The model under review builds one solid part; all positions refer to its coordinate system, in mm. Face numbers are marked on the shaded views. Coordinates: 2 decimals unless noted, no trailing zeros. Order: outer loops, then holes, each group sorted by start corner. A loop starts at its lowest first (then second) coordinate and runs counter-clockwise, first axis right, second up. Notation, with made-up numbers: (61.5, -17.5) -> (66.5, -17.5) arc R5 ccw to (66.5, -10.5) -> close; hole circle Ø9 at (-29.75, 88.5). An arc over 180 degrees is marked (long way). Put each result on its own line as item: value.
Autodesk Inventor part; units mm, degrees
ref_plane "YZ Plane" through (0, 0, 0) normal (1, 0, 0) x (0, 1, 0)
ref_plane "XZ Plane" through (0, 0, 0) normal (0, 1, 0) x (-1, 0, 0)
ref_plane "XY Plane" through (0, 0, 0) normal (0, 0, 1) x (1, 0, 0)
sketch "Sketch1" plane through (0, 0, 0) normal (0, 1, 0) x (-1, 0, 0)
  line L0 (243.2455, 20) -> (-243.2455, 20)
  line L1 (-243.2455, 20) -> (-243.2455, -20)
  line L2 (-243.2455, -20) -> (243.2455, -20)
  line L3 (243.2455, -20) -> (243.2455, 20)
  line L4 (243.2455, 20) -> (-243.2455, -20) construction
  line L5 (-243.2455, 20) -> (243.2455, -20) construction
  line L6 (243.2455, 35) -> (-258.2455, 35)
  line L7 (-258.2455, 35) -> (-258.2455, -35)
  line L8 (-258.2455, -35) -> (243.2455, -35)
  line L9 (243.2455, -35) -> (243.2455, 35)
  line L10 (243.2455, 35) -> (-258.2455, -35) construction
  line L11 (-258.2455, 35) -> (243.2455, -35) construction
  point P0 (0, 0)
  point P1 (-7.5, 0)
  point P2 (243.2455, 20)
  point P3 (243.2455, -20)
  dimension "d0" = 486.491
  dimension "d1" = 40
  dimension "d2" = 15
  dimension "d3" = 15
extrude "Extrusion1" add sketch "Sketch1" along normal blind 15 contours L3 L2 L1 L0
extrude "Extrusion2" add sketch "Sketch1" along normal blind 25 contours L0 L1 L2 L9 L8 L7 L6
fillet "Fillet1" radius 24 2 edges at (258.2455, 12.5, -35) (258.2455, 12.5, 35)
fillet "Fillet2" radius 5 11 edges at (258.2455, 0, 0) (-4.5, 0, 35) (-4.5, 0, -35) (-243.2455, 12.5, -35) (-243.2455, 12.5, 35) (251.2161, 25, -27.9706) (258.2455, 25, 0) (251.2161, 25, 27.9706) (-4.5, 25, 35) (-4.5, 25, -35) (-243.2455, 0, 0)
properties part number "ArmRestCushion"
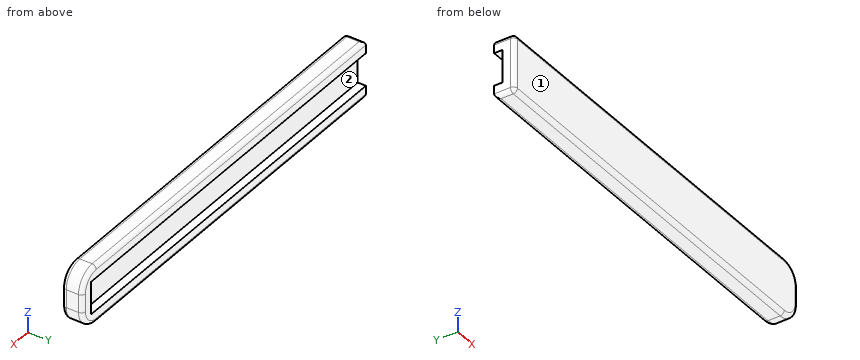
Item 1: For line 1 (Z direction, x = 90, y = 17); line 2 (Y direction, x = 116, z = -16.5); line 3 (Z direction, x = -175.5, y = 21.5), list the stretches that pass through material, from the lowest coordinate up. Write a range as from..to.
Answers below:
line 1: -35..-20, 20..35
line 2: 0..15
line 3: -34.77..-20, 20..34.77
Item 2: Consider section B-B on z = 6. Write out the cut boundary in (x, y), and give its area (3 significant figures).
Answers below:
outline: (-243.25, 5) arc R5 ccw to (-238.25, 0) -> (253.25, 0) arc R5 ccw to (258.25, 5) -> (258.25, 20) arc R5 ccw to (253.25, 25) -> (243.25, 25) -> (243.25, 15) -> (-243.25, 15) -> close
area: 7,660 mm^2
Item 3: For pin 1 Ø5 at (y, z) = (21.5, -1.5) entering from -X; pin 2 Ø6 at (y, z) = (22, -14.5) entering from +X; pin 3 Ø5 at (x, z) = (188.5, 17) entering from +Y, all flat-tipped, find the tip position at first contact; note any pin that passes through.
Answers below:
pin 1: x = 243.25
pin 2: x = 258.22
pin 3: y = 15
Item 4: Mouldability with a two-part tool opening along Z and no side actions: class the marked faces 1 and 2 as +Z half, -Z half, draft (parallel to the pull), parting line (faces both ways), or undercut.
Answers below:
face 1: draft
face 2: undercut
Item 5: Consider section A-A on x = 224. Write out the cut boundary in (y, z).
Answers below:
outline: (0, -30) arc R5 ccw to (5, -35) -> (20, -35) arc R5 ccw to (25, -30) -> (25, -20) -> (15, -20) -> (15, 20) -> (25, 20) -> (25, 30) arc R5 ccw to (20, 35) -> (5, 35) arc R5 ccw to (0, 30) -> close
